Read the model definition and answer for the solid it produces. Units are mm, in the model's axes. A direction names the side the tool comes from. Round coordinates to 2 decimals unless told otherwise and drop trailing zeros. Order: outer loops, then holes, each group sorted by start corner. A loop starts at its lowest first (then second) coordinate and runs counter-clockwise, first axis right, second up. Notation, with made-up numbers: (69, 21) -> (85, 21) arc R5 ccw to (85, 27) -> close; hole circle Ø7 at (80.5, 41). An arc over 180 degrees is marked (long way). Answer as a JSON object with one key per item and string values. Group by question number.
Item 1: Section B-B, the plane x = 6 is taken. Write down the section's boundary in (y, z) (3 decimals), plus the area to 3 significant figures.
Item 2: Section A-A, the plane y = -147.5 is taken. Write down the section's boundary in (x, z) (3 decimals), plus the area to 3 significant figures.
Item 3: Section D-D, the plane y = -312 is taken. Write down the section's boundary in (x, z) (3 decimals), plus the area to 3 significant figures.
Item 4: Consider probe 1 along Z at (x, y) = (1, -197) (3 decimals); probe 2 along Y at (x, z) = (8, 87.5) (3 decimals); probe 3 along Z at (x, y) = (1, -108) (3 decimals). Determine where each line is inside the solid, lowest interval first. Write a range as from..to.
Item 5: For faces 1 (the flat face through (4.7, -221.77, 417.11)), 2 (the flat face through (4.696, -183.143, 320.761)), determine the directions among +Z, -Z, +X, -X, +Y, -Y from which every point of the face is accessible in a straight line to the end or side of a thin tool.
Item 6: Section C-C, the plane z = 75.5 is taken. Write down the section's boundary in (x, y) (3 decimals).
Item 7: Given P1, Ø5, axis at x = 8.5, z = 476.5, coming from the -Y side (3 decimals); P2, Ø2, axis at x = 8.5, z = 468, coming from the +Y side; P3, Ø1, axis at x = 1.5, y = -232.5, coming from the +Z side, each flat-ended and moving along its own axis, determine where each tip first touches the part or whether it passes through.
from build123d import *

# Parameters (mm, degrees)
F1_DEPTH = 9.525


with BuildPart() as f1:
    # F0 (on Right) → F1 (new body)
    with BuildSketch(Plane.YZ):
        Polygon((-76.2, 546.145316), (-76.2, 723.9), (-371.475, 101.6), (-287.132216, 101.6), align=None)
        Polygon((-177.8, 9.525), (-85.725, 9.525), (-85.725, 101.6), (-287.132216, 101.6), (-371.475, 101.6), (-371.475, 9.525), (-279.4, 9.525), align=None)
    extrude(amount=F1_DEPTH)


solid = f1.part
Values found:
{
 "1": {"outline": "(-371.475, 9.525) -> (-85.725, 9.525) -> (-85.725, 101.6) -> (-287.132, 101.6) -> (-76.2, 546.145) -> (-76.2, 723.9) -> (-371.475, 101.6) -> close", "area": "71,300 mm2"},
 "2": {"outline": "(0, 9.525) -> (9.525, 9.525) -> (9.525, 101.6) -> (0, 101.6) -> close; (0, 395.879) -> (9.525, 395.879) -> (9.525, 573.633) -> (0, 573.633) -> close", "area": "2,570 mm2"},
 "3": {"outline": "(0, 9.525) -> (9.525, 9.525) -> (9.525, 226.945) -> (0, 226.945) -> close", "area": "2,070 mm2"},
 "4": {"probe 1": "9.525..101.6, 291.556..469.311", "probe 2": "-371.475..-85.725", "probe 3": "9.525..101.6, 479.126..656.881"},
 "5": {"face 1": "+Z, +X, -X, -Y", "face 2": "+X, -X, +Y"},
 "6": {"outline": "(0, -371.475) -> (9.525, -371.475) -> (9.525, -85.725) -> (0, -85.725) -> close"},
 "7": {"P1": "y = -194.775", "P2": "y = -112.8", "P3": "z = 395.55"}
}
